Autodesk Inventor part; units mm, degrees
ref_plane "YZ Plane" through (0, 0, 0) normal (1, 0, 0) x (0, 1, 0)
ref_plane "XZ Plane" through (0, 0, 0) normal (0, 1, 0) x (-1, 0, 0)
ref_plane "XY Plane" through (0, 0, 0) normal (0, 0, 1) x (1, 0, 0)
sketch "Sketch1" plane through (0, 0, 0) normal (0, 1, 0) x (-1, 0, 0)
  line L0 (0, 0) -> (9.75, 0)
  line L1 (9.75, 0) -> (9.75, -9.75)
  line L2 (9.75, -9.75) -> (0, -9.75)
  line L3 (0, -9.75) -> (0, 0)
  dimension "d0" = 9.75
  dimension "d1" = 9.75
extrude "Extrusion1" add sketch "Sketch1" along normal blind 5
sketch "Sketch2" plane through (0, 5, 0) normal (0, 1, 0) x (1, 0, 0)
  line L0 (0, 9.75) -> (-9.75, 9.75)
  line L1 (-9.75, 9.75) -> (-9.75, 0)
  line L2 (-9.75, 0) -> (0, 0)
  line L3 (0, 0) -> (0, 9.75)
  circle A0 centre (-4.875, 4.875) radius 1.8
  dimension "d4" = 3.6
extrude "Extrusion2" add sketch "Sketch2" along normal blind 3 contours A0
sketch "Sketch3" plane through (-4.875, 8, -4.875) normal (0, 1, 0) x (1, 0, 0)
  circle A0 centre (0, 0) radius 1.8
  line L0 (-0.5, -2.1786) -> (0.5, -2.1786)
  line L1 (0.5, -2.1786) -> (0.5, 2.1786)
  line L2 (0.5, 2.1786) -> (-0.5, 2.1786)
  line L3 (-0.5, 2.1786) -> (-0.5, -2.1786)
  line L4 (-0.5, -2.1786) -> (0.5, 2.1786) construction
  line L5 (0.5, -2.1786) -> (-0.5, 2.1786) construction
  point P0 (4.875, -4.875)
  point P1 (-0.5, 1.7292)
  point P2 (-0.5, -1.7292)
  point P3 (0.5, -1.7292)
  point P4 (0.5, 1.7292)
  dimension "d7" = 1
extrude "Extrusion3" cut sketch "Sketch3" against normal blind 3 contours L1 A0 L3
properties part number "Pot"
Work out the finished part from the listing and answer in its coordinate system (mm). A direction names the side the tool comes from. Give positions to 0.01 mm unless a question says otherwise; leave off trailing zeros. Order: outer loops, then holes, each group sorted by start corner. A loop starts at its lowest first (then second) coordinate and runs counter-clockwise, first axis right, second up. Notation, with made-up numbers: (5.25, 13.25) -> (50.25, 13.25) arc R26 ccw to (50.25, 32.25) -> close; hole circle Ø9 at (38.25, 50). An arc over 180 degrees is marked (long way). One line per item, written item: value.
Item 1: Find section A-A, the plane y = 6.75. Give the vertices of the cut face in (x, z) (3 decimals), plus the area to 3 significant figures.
Answer sheet:
outline: (-5.375, -6.604) -> (-5.375, -3.146) arc R1.8 ccw to start; (-4.375, -6.604) arc R1.8 ccw to (-4.375, -3.146) -> close
area: 6.63 mm²
Item 2: Determine the mould class of faces 1 (the flat face through (-6, 8, -5)), 2 (the cylindrical face through (-3.075, 6.479, -4.907)), 3 (the flat face through (-5.375, 7, -5)) for opening direction X: released by +X, released by -X, zero draft, split by the parting line, or undercut.
Answer sheet:
face 1: zero draft
face 2: released by +X
face 3: undercut
Item 3: Find section C-C, the plane x = -8. Give the vertices of the cut face in (y, z).
Answer sheet:
outline: (0, -9.75) -> (5, -9.75) -> (5, 0) -> (0, 0) -> close
Item 4: Flat-ended cylindrical pins translate along their axes: P1, Ø1.5, axis at x = -8.5, z = -6.5, coming from the +Y side; P2, Ø0.9, axis at y = 6, z = -5.5, coming from the +X side; P3, Ø0.9, axis at y = 7, z = -5.5, coming from the -X side. Find the tip coordinate at first contact, or state that the pin passes through.
Answer sheet:
P1: y = 5
P2: x = -3.08
P3: x = -6.67
Item 5: Straight lines are drawn through the part: probe 1 along Y at (x, z) = (-1.75, -1); probe 2 along X at (y, z) = (6, -3.5) (3 decimals); probe 3 along Z at (x, y) = (-6, 6.5). For each, find the intervals that lie inside material, in ascending order.
Answer sheet:
probe 1: 0 to 5
probe 2: -6.037 to -5.375, -4.375 to -3.713
probe 3: -6.28 to -3.47
Item 6: Find section B-B, the plane z = -5. Give the vertices of the cut face in (x, y) (3 decimals).
Answer sheet:
outline: (-9.75, 0) -> (0, 0) -> (0, 5) -> (-3.079, 5) -> (-3.079, 8) -> (-4.375, 8) -> (-4.375, 5) -> (-5.375, 5) -> (-5.375, 8) -> (-6.671, 8) -> (-6.671, 5) -> (-9.75, 5) -> close
Item 7: Find section D-D, the plane z = -2.75. Give the vertices of the cut face in (x, y).
Answer sheet:
outline: (-9.75, 0) -> (0, 0) -> (0, 5) -> (-9.75, 5) -> close
Item 8: A tool of negligible diameter and unlimited length cuts with its end or side. For faces 4 (the flat face through (-4.375, 7, -5)), 5 (the cylindrical face through (-6.675, 6.479, -4.843)), 6 (the flat face through (-5, 0, -5)), from which of +Z, -Z, +X, -X, +Y, -Y can it reach the whole face along a straight path? Write none if from no direction.
Answer sheet:
face 4: +Z, -Z, +Y
face 5: -X, +Y
face 6: +Z, -Z, +X, -X, -Y
